Input: dimensioned drawing with shaded views. Units: mm. Origin: part minimum x, y, z. Coordinates: 2 decimals unless noted, no trailing zeros. Answer as CSV lines item,"result".
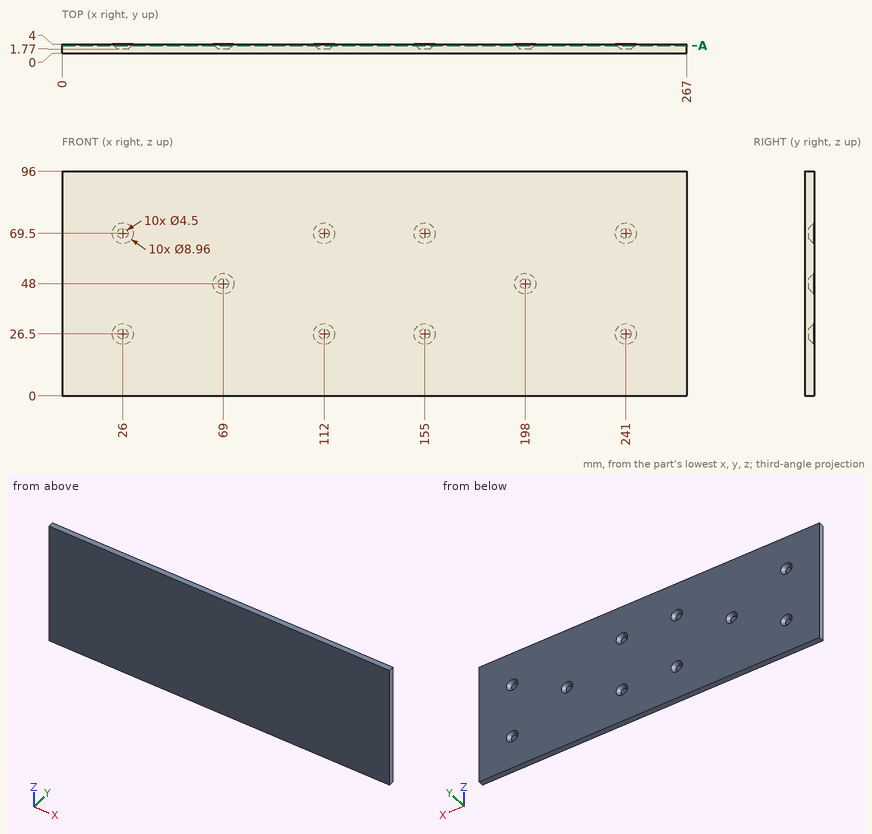
1. Cut plane A-A (y = 3.35). State how many separate pieces and enclosed holes the cut face has, plus the area to 3 significant figures.
Findings:
separate pieces,"1"
enclosed holes,"10"
area,"25,200 mm2"
2. Contact query for flat-ended pins moving along their axis: pin 1 (3.5 mm diameter, centred on x = 70, z = 48.5, fed in from +Y); pin 2 (2 mm diameter, centred on x = 156, z = 27.5, fed in from +Y); pin 3 (2 mm diameter, centred on x = 199, z = 47.5, fed in from +Y). Output: stop coordinate, or through.
Findings:
pin 1,"stops at y = 2.39"
pin 2,"stops at y = 1.93"
pin 3,"stops at y = 1.77"
3. Ray query, line 1 along X through (y, z) = (2.9, 48); line 2 along Z through (x, y) = (68, 3.25); line 3 along X through (y, z) = (2.4, 69). Return the intervals inside material, ascending.
Findings:
line 1,"x = 0 to 65.62, 72.38 to 194.62, 201.38 to 267"
line 2,"z = 0 to 44.41, 51.59 to 96"
line 3,"x = 0 to 23.16, 28.84 to 109.16, 114.84 to 152.16, 157.84 to 238.16, 243.84 to 267"
